Can you work these out from the model? Positions are in its coordinate system, mm. Face numbers are marked on the shaded views. A direction names the side the tool comes from. Round coordinates to 2 decimals unless told otherwise and drop trailing zeros. Loops run counter-clockwise (first coordinate to the right, second up) from the corner with the lowest first, then second, coordinate; pieces in that order, holes last. Notation, with made-up numbers: (-2, 47.25) -> (12, 47.25) arc R7 ccw to (12, 54.25) -> close; hole circle Ø4 at (42, -19.5). An arc over 180 degrees is marked (long way). Write each question's results on one line, items separated by ' | '.
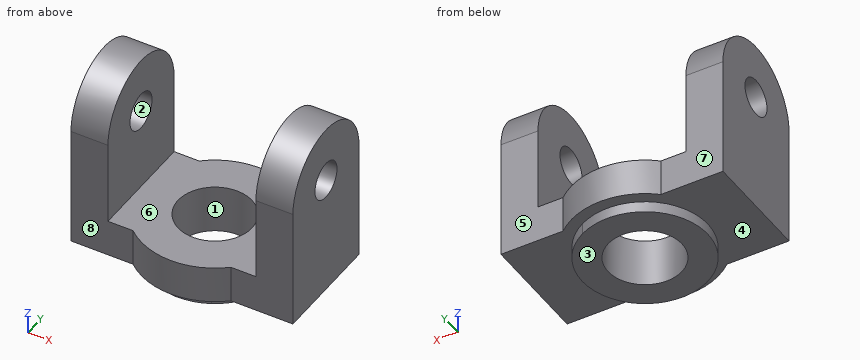
from build123d import *

# Parameters (mm, degrees)
F0_R     = 10
F1_DEPTH = 10
F2_DEPTH = 3
F3_W     = 10
F3_H     = 30
F4_DEPTH = 38
F5_R     = 5
F6_DEPTH = 75
F8_DEPTH = 75


with BuildPart() as f1:
    # F0 (on Top) → F1 (new body)
    with BuildSketch(Plane.XY):
        with BuildLine():
            ThreePointArc((13.2287565553, 15), (18.2287565553, 8.2287565553), (20, 0))
            ThreePointArc((20, 0), (18.2287565553, -8.2287565553), (13.2287565553, -15))
            Line((13.2287565553, -15), (30, -15))
            Line((30, -15), (30, 15))
            Line((30, 15), (13.2287565553, 15))
        make_face()
        with BuildLine():
            ThreePointArc((-13.2287565553, -15), (-20, 0), (-13.2287565553, 15))
            Line((-13.2287565553, 15), (-30, 15))
            Line((-30, 15), (-30, -15))
            Line((-30, -15), (-13.2287565553, -15))
        make_face()
        with BuildLine():
            Line((8, 15), (13.2287565553, 15))
            ThreePointArc((13.2287565553, 15), (0, 20), (-13.2287565553, 15))
            Line((-13.2287565553, 15), (-8, 15))
            ThreePointArc((-8, 15), (0, 17), (8, 15))
        make_face()
        with BuildLine():
            ThreePointArc((-13.2287565553, -15), (0, -20), (13.2287565553, -15))
            Line((13.2287565553, -15), (8, -15))
            ThreePointArc((8, -15), (0, -17), (-8, -15))
            Line((-8, -15), (-13.2287565553, -15))
        make_face()
        with BuildLine():
            ThreePointArc((13.2287565553, -15), (18.2287565553, -8.2287565553), (20, 0))
            ThreePointArc((20, 0), (18.2287565553, 8.2287565553), (13.2287565553, 15))
            Line((13.2287565553, 15), (8, 15))
            ThreePointArc((8, 15), (14.5773797371, 8.7464278423), (17, 0))
            ThreePointArc((17, 0), (14.5773797371, -8.7464278423), (8, -15))
            Line((8, -15), (13.2287565553, -15))
        make_face()
        with BuildLine():
            Line((-8, 15), (-13.2287565553, 15))
            ThreePointArc((-13.2287565553, 15), (-20, 0), (-13.2287565553, -15))
            Line((-13.2287565553, -15), (-8, -15))
            ThreePointArc((-8, -15), (-17, 0), (-8, 15))
        make_face()
        with BuildLine():
            ThreePointArc((17, 0), (14.5773797371, 8.7464278423), (8, 15))
            Line((8, 15), (-8, 15))
            ThreePointArc((-8, 15), (-17, 0), (-8, -15))
            Line((-8, -15), (8, -15))
            ThreePointArc((8, -15), (14.5773797371, -8.7464278423), (17, 0))
        make_face()
        Circle(F0_R, mode=Mode.SUBTRACT)
        with BuildLine():
            Line((-8, 15), (8, 15))
            ThreePointArc((8, 15), (0, 17), (-8, 15))
        make_face()
        with BuildLine():
            ThreePointArc((-8, -15), (0, -17), (8, -15))
            Line((8, -15), (-8, -15))
        make_face()
    extrude(amount=F1_DEPTH)

    # F0 (on Top) → F2 (join)
    with BuildSketch(Plane.XY):
        with BuildLine():
            ThreePointArc((17, 0), (14.5773797371, 8.7464278423), (8, 15))
            Line((8, 15), (-8, 15))
            ThreePointArc((-8, 15), (-17, 0), (-8, -15))
            Line((-8, -15), (8, -15))
            ThreePointArc((8, -15), (14.5773797371, -8.7464278423), (17, 0))
        make_face()
        Circle(F0_R, mode=Mode.SUBTRACT)
        with BuildLine():
            ThreePointArc((-8, -15), (0, -17), (8, -15))
            Line((8, -15), (-8, -15))
        make_face()
        with BuildLine():
            Line((-8, 15), (8, 15))
            ThreePointArc((8, 15), (0, 17), (-8, 15))
        make_face()
    extrude(amount=-F2_DEPTH)

    # F3 (on face) → F4 (join)
    with BuildSketch(Plane.XY.offset(10)):
        with Locations((-25, 0)):
            Rectangle(F3_W, F3_H)
        with Locations((25, 0)):
            Rectangle(F3_W, F3_H)
    extrude(amount=F4_DEPTH)

    # F5 (on face) → F6 (cut)
    with BuildSketch(Plane.YZ.offset(30)):
        with Locations((0, 32.5)):
            Circle(F5_R)
    extrude(amount=-F6_DEPTH, mode=Mode.SUBTRACT)

    # F7 (on face) → F8 (cut)
    with BuildSketch(Plane.YZ.offset(30)):
        with BuildLine():
            Line((-15, 48), (-15, 32.675947994))
            ThreePointArc((-15, 32.675947994), (0, 47.5010318877), (15, 32.675947994))
            Line((15, 32.675947994), (15, 48))
            Line((15, 48), (-15, 48))
        make_face()
    extrude(amount=-F8_DEPTH, mode=Mode.SUBTRACT)


solid = f1.part
1. Will these pins go through, and if not, where does the flat tip stop? pin 1 (20 mm diameter, centred on x = 3.5, y = 0.5, fed in from +Z); pin 2 (3 mm diameter, centred on x = 21, z = 6.5, fed in from +Y); pin 3 (6 mm diameter, centred on x = 21.5, y = 14, fed in from +Z).
Final values:
pin 1: z = 10 | pin 2: y = 15 | pin 3: z = 42.7
2. We'd pull the mould along Z, two halves only. Please class the marked faces 1, 2 and 3: pulls with the +Z half, pulls with the -Z half, needs draft (parallel to the pull), parting line crosses it, or undercut.
Final values:
face 1: needs draft | face 2: undercut | face 3: pulls with the -Z half
3. If we section it at A-A (x = 0): List the corners of the cut face in (y, z) for me, then the cut area to 3 significant figures.
Final values:
outline: (-20, 0) -> (-17, 0) -> (-17, -3) -> (-10, -3) -> (-10, 10) -> (-20, 10) -> close; (10, -3) -> (17, -3) -> (17, 0) -> (20, 0) -> (20, 10) -> (10, 10) -> close | area: 242 mm2
4. If we section it at D-D (x = 25.5): List the corners of the cut face in (y, z) for me, then the cut area to 3 significant figures.
Final values:
outline: (-15, 0) -> (15, 0) -> (15, 32.68) arc R15 ccw to (-15, 32.68) -> close; hole circle Ø10 at (0, 32.5) | area: 1,250 mm2
5. On a 3-axis mill with a long thin cutter (end or side, diameter ignored), from which of +Z, -Z, +X, -X, +Y, -Y can I reach the whole of each face in a straight line? I mean the marked faces 4, 5, 6, 7 and 8. Say none if no direction works.
Final values:
face 4: -Z | face 5: +Z, -Z, +X, +Y | face 6: +Z, +Y, -Y | face 7: +Z, -Z, -X, +Y | face 8: +Z, -Z, -X, -Y
6. Please list where these lines run through material, in increasing order: line 1 (Y direction, x = 0, z = 6); line 2 (X direction, y = -9, z = 31.5); line 3 (Y direction, x = 13.5, z = 1). Write a range as from..to.
Final values:
line 1: -20..-10, 10..20 | line 2: -30..-20, 20..30 | line 3: -15..15
7. If we section it at C-C (y = 2): List the corners of the cut face in (x, z) for me.
Final values:
outline: (-30, 0) -> (-16.88, 0) -> (-16.88, -3) -> (-9.8, -3) -> (-9.8, 10) -> (-20, 10) -> (-20, 27.92) -> (-30, 27.92) -> close; (-30, 37.08) -> (-20, 37.08) -> (-20, 47.37) -> (-30, 47.37) -> close; (9.8, -3) -> (16.88, -3) -> (16.88, 0) -> (30, 0) -> (30, 27.92) -> (20, 27.92) -> (20, 10) -> (9.8, 10) -> close; (20, 37.08) -> (30, 37.08) -> (30, 47.37) -> (20, 47.37) -> close
8. If we section it at B-B (z = 2): List the corners of the cut face in (x, y) for me, then the cut area to 3 significant figures.
Final values:
outline: (-30, -15) -> (-13.23, -15) arc R20 ccw to (13.23, -15) -> (30, -15) -> (30, 15) -> (13.23, 15) arc R20 ccw to (-13.23, 15) -> (-30, 15) -> close; hole circle Ø20 at (0, 0) | area: 1,670 mm2
